The listing builds one solid part. Answer for the finished solid, in the listing's coordinates (mm). A direction names the side the tool comes from. Coordinates: 2 decimals unless noted, no trailing zeros. Order: outer loops, then holes, each group sorted by start corner. A loop starts at its lowest first (then second) coordinate and runs counter-clockwise, first axis right, second up.
from build123d import *

# Parameters (mm, degrees)
SKETCH1_W           = 72
SKETCH1_H           = 27
BOSS_EXTRUDE1_DEPTH = 6
SKETCH2_W           = 12
SKETCH2_H           = 15
CUT_EXTRUDE1_DEPTH  = 78.129760793
SKETCH3_W           = 8
SKETCH3_H           = 14
BOSS_EXTRUDE2_DEPTH = 4
CUT_EXTRUDE2_DEPTH  = 78.129760793
SKETCH5_W           = 12
SKETCH5_H           = 6
BOSS_EXTRUDE3_DEPTH = 4
CUT_EXTRUDE4_DEPTH  = 78.129760793
SKETCH8_R           = 2.15
CUT_EXTRUDE5_DEPTH  = 10
SKETCH9_R           = 1.45
CUT_EXTRUDE6_DEPTH  = 78.129760793
FILLET2_R           = 4


with BuildPart() as part:
    # Sketch1 → Boss-Extrude1 (new body)
    with BuildSketch(Plane(origin=(0, 0, 0), x_dir=(1, 0, 0), z_dir=(0, 1, 0))):
        with Locations((36, -13.5)):
            Rectangle(SKETCH1_W, SKETCH1_H)
    extrude(amount=BOSS_EXTRUDE1_DEPTH)

    # Sketch2 → Cut-Extrude1 (cut, through all)
    with BuildSketch(Plane(origin=(0, 6, 0), x_dir=(1, 0, 0), z_dir=(0, 1, 0))):
        with Locations((6, -13.5)):
            Rectangle(SKETCH2_W, SKETCH2_H)
    extrude(amount=-CUT_EXTRUDE1_DEPTH, mode=Mode.SUBTRACT)

    # Sketch3 → Boss-Extrude2 (add)
    with BuildSketch(Plane(origin=(0, 0, 0), x_dir=(-1, 0, 0), z_dir=(0, -1, 0))):
        with Locations((-68, -13.5)):
            Rectangle(SKETCH3_W, SKETCH3_H)
    extrude(amount=BOSS_EXTRUDE2_DEPTH)

    # Sketch4 → Cut-Extrude2 (cut, through all)
    with BuildSketch(Plane(origin=(0, 0, 0), x_dir=(-1, 0, 0), z_dir=(0, -1, 0))):
        Polygon((-64, -20.5), (-22, -27), (-72, -27), (-72, -20.5), align=None)
        Polygon((-64, -6.5), (-22, 0), (-72, 0), (-72, -6.5), align=None)
    extrude(amount=-CUT_EXTRUDE2_DEPTH, mode=Mode.SUBTRACT)

    # Sketch5 → Boss-Extrude3 (add)
    with BuildSketch(Plane.XZ):
        with Locations((6, 3)):
            Rectangle(SKETCH5_W, SKETCH5_H)
        with Locations((6, 24)):
            Rectangle(SKETCH5_W, SKETCH5_H)
    extrude(amount=BOSS_EXTRUDE3_DEPTH)

    # Sketch7 → Cut-Extrude4 (cut, through all)
    with BuildSketch(Plane(origin=(0, 0, 0), x_dir=(-1, 0, 0), z_dir=(0, -1, 0))):
        Polygon((-18.5, -20.5), (-18.5, -6.5), (-64, -10.5), (-64, -16.5), align=None)
    extrude(amount=-CUT_EXTRUDE4_DEPTH, mode=Mode.SUBTRACT)

    # Sketch8 → Cut-Extrude5 (cut)
    with BuildSketch(Plane(origin=(72, 0, 0), x_dir=(0, 0, -1), z_dir=(1, 0, 0))):
        with Locations((-13.5, 1)):
            Circle(SKETCH8_R)
    extrude(amount=-CUT_EXTRUDE5_DEPTH, mode=Mode.SUBTRACT)

    # Sketch9 → Cut-Extrude6 (cut, through all)
    with BuildSketch(Plane(origin=(0, 0, 0), x_dir=(-1, 0, 0), z_dir=(0, 0, -1))):
        with Locations((-5, 1)):
            Circle(SKETCH9_R)
    extrude(amount=-CUT_EXTRUDE6_DEPTH, mode=Mode.SUBTRACT)

    # Fillet2
    # the kernel refuses this fillet: 4 mm, written as the material it takes off along each edge
    with BuildSketch(Plane(origin=(0, -4, 11), x_dir=(0, 1, 0), z_dir=(0, 0, 1)), Plane(origin=(0, -4, 16), x_dir=(1, 0, 0), z_dir=(0, 0, -1)), Plane(origin=(12, -4, 37), x_dir=(0, 1, 0), z_dir=(0, 0, -1))) as fillet2_piece_1:
        with BuildLine():
            CenterArc((FILLET2_R, -FILLET2_R), FILLET2_R, 90, 90)
            Line((0, -FILLET2_R), (0, 0))
            Line((0, 0), (FILLET2_R, 0))
        make_face()
    extrude(amount=26, mode=Mode.SUBTRACT)
    with BuildSketch(Plane(origin=(12, -4, -10), x_dir=(0, 1, 0), z_dir=(0, 0, 1))) as fillet2_piece_2:
        with BuildLine():
            CenterArc((FILLET2_R, FILLET2_R), FILLET2_R, 180, 90)
            Line((0, FILLET2_R), (0, 0))
            Line((0, 0), (FILLET2_R, 0))
        make_face()
    extrude(amount=26, mode=Mode.SUBTRACT)
    with BuildSketch(Plane(origin=(72, -4, -3.5), x_dir=(0, 1, 0), z_dir=(0, 0, 1)), Plane(origin=(64, -4, 30.5), x_dir=(0, 1, 0), z_dir=(0, 0, -1))) as fillet2_piece_3:
        with BuildLine():
            CenterArc((FILLET2_R, FILLET2_R), FILLET2_R, 180, 90)
            Line((0, FILLET2_R), (0, 0))
            Line((0, 0), (FILLET2_R, 0))
        make_face()
    extrude(amount=34, mode=Mode.SUBTRACT)


solid = part.part
1) Determine the mould class of faces 4 (the face through (41.57, 2.96, 18.47)), 5 (the face through (6, -4, 3)), 6 (the face through (68.06, 1.65, 11.45)) for opening direction Y: released by +Y, released by -Y, zero draft, split by the parting line, or undercut.
2) Section C-C (z = 23.25) is taken. Give the vertices of the cut face in (x, y), then the cut area to 3 significant figures.
3) Section B-B (x = 5) is taken. Give the vertices of the cut face in (y, z).
4) Section D-D (z = 8) is taken. Give the vertices of the cut face in (x, y).
5) Section A-A (y = 1) is taken. Give the vertices of the cut face in (x, z).
6) Each of these flat-tipped pins is pushed along its axis until it touches: P1, Ø6, axis at x = 38.5, y = -1.5, coming from the +Z side; P2, Ø3, axis at x = 47.5, y = 1, coming from the +Z side; P3, Ø4, axis at x = 66.5, y = 3, coming from the -Z side. Where does it stop, or does it pass through?
7) A tool of negligible diameter and unlimited length cuts with its end or side. For faces 1 (the face through (32, 0, 7)), 2 (the face through (40.93, 2.96, 8.47)), 3 (the face through (68, 1, 6.5)), from which of +Z, -Z, +X, -X, +Y, -Y can it reach the whole face along a straight path? Write none if from no direction.
8) Consider L1, parallel to Y at x = 5, z = 22.5; L2, parallel to Z at x = 9, y = 4.75; L3, parallel to X at y = 3.25, z = 15.5. Determine where each line is inside the solid, lowest interval first.
Filled sheet:
1. face 4: zero draft
1. face 5: released by -Y
1. face 6: undercut
2. outline: (0, 0) arc R4 ccw to (4, -4) - (8, -4) arc R4 ccw to (12, 0) - (46.23, 0) - (46.23, 6) - (0, 6) - close; hole circle Ø2.9 at (5, 1)
2. area: 312 mm2
3. outline: (-4, 0) - (-0.45, 0) - (-0.45, 6) - (-4, 6) - close; (-4, 21) - (-0.45, 21) - (-0.45, 27) - (-4, 27) - close; (2.45, 0) - (6, 0) - (6, 6) - (2.45, 6) - close; (2.45, 21) - (6, 21) - (6, 27) - (2.45, 27) - close
4. outline: (12, 0) - (18.5, 0) - (18.5, 6) - (12, 6) - close; (35.56, 0) - (64, 0) arc R4 ccw to (72, 0) - (72, 6) - (35.56, 6) - close
5. outline: (0, 0) - (3.55, 0) - (3.55, 6) - (0, 6) - close; (0, 21) - (3.55, 21) - (3.55, 27) - (0, 27) - close; (6.45, 0) - (22, 0) - (64, 6.5) - (72, 6.5) - (72, 11.35) - (64, 11.35) - (64, 10.5) - (18.5, 6.5) - (18.5, 20.5) - (64, 16.5) - (64, 15.65) - (72, 15.65) - (72, 20.5) - (64, 20.5) - (22, 27) - (6.45, 27) - (6.45, 21) - (12, 21) - (12, 6) - (6.45, 6) - close
6. P1: stops at z = 24.85
6. P2: stops at z = 23.29
6. P3: stops at z = 6.5
7. face 1: +Z, -Z, -Y
7. face 2: +Y, -Y
7. face 3: -Z, +X, +Y, -Y
8. L1: y = -4 to -0.45, 2.45 to 6
8. L2: z = 0 to 6, 21 to 27
8. L3: x = 12 to 18.5, 64 to 72
